For this review, take the finished solid that the model builds, in its own axes (mm). A direction names the side the tool comes from. Coordinates: 2 decimals unless noted, no trailing zeros. Order: outer loops, then holes, each group sorted by start corner. A loop starts at its lowest first (then second) coordinate and runs counter-clockwise, first axis right, second up.
Autodesk Inventor part; units mm, degrees
ref_plane "YZ Plane" through (0, 0, 0) normal (1, 0, 0) x (0, 1, 0)
ref_plane "XZ Plane" through (0, 0, 0) normal (0, 1, 0) x (-1, 0, 0)
ref_plane "XY Plane" through (0, 0, 0) normal (0, 0, 1) x (1, 0, 0)
sketch "Sketch1" plane through (0, 0, 0) normal (0, 1, 0) x (-1, 0, 0)
  line L0 (0, 74.2932) -> (20.6375, 74.2932)
  line L1 (20.6375, 74.2932) -> (20.6375, 45.7421)
  line L2 (13.589, 67.9432) -> (0, 67.9432)
  line L3 (16.6624, -52.7068) -> (20.6375, -52.7068)
  line L4 (20.6375, -52.7068) -> (20.6375, 45.7421)
  line L5 (16.6624, -52.7068) -> (16.6624, -78.1068)
  line L6 (16.6624, -78.1068) -> (13.589, -78.1068)
  line L7 (13.589, -78.1068) -> (13.589, 67.9432)
  line L8 (0, 68.4776) -> (0, -51.9613) construction
  line L9 (13.589, 67.9432) -> (13.589, 74.2932)
  point P0 (0, 0)
  dimension "d0" = 20.6375
  dimension "d1" = 127
  dimension "d2" = 6.35
  dimension "d3" = 16.6624
  dimension "d4" = 13.589
  dimension "d12" = 25.4
  dimension "d19" = 3.0734
revolve "Revolution1" add sketch "Sketch1" angle 360 about axis through (0, 0, 68.4776) along (0, 0, -1)
thread "Thread1"
chamfer "Chamfer2" distance 1.27 angle 45 1 edges at (20.6375, 0, -52.7068)
chamfer "Chamfer3" distance 1.27 angle 45 1 edges at (20.6375, 0, 74.2932)
properties part number "EndHilt" material "Aluminum 6061"
1. To check wall thickness, follow L1, parallel to Y at x = 0, z = 0.5; L2, parallel to Z at x = 11, y = 14; L3, parallel to X at y = 6, z = -23.5. State the ranges of each line that lie inside material, in increasing order.
Answer below:
L1: y = -20.64 to -13.59, 13.59 to 20.64
L2: z = -52.71 to 74.29
L3: x = -19.75 to -12.19, 12.19 to 19.75
2. The part is to be moulded in two halves that separate along Y. For faces 1 (the face through (4.474, -20.147, 9.922)), 2 (the face through (14, 0, -78.107)), 3 (the face through (-12.96, -4.08, -0.84)), say which applies: +Y half, -Y half, draft (parallel to the pull), parting line (faces both ways), or undercut.
Answer below:
face 1: parting line
face 2: draft
face 3: undercut
3. Clearance check with flat-ended pins moving along their axes: pin 1 Ø3 at (y, z) = (4.5, 52) entering from -X; pin 2 Ø1 at (x, z) = (2.5, 11.5) entering from -Y; pin 3 Ø1.5 at (y, z) = (-7.5, -32) entering from -X. State where each tip first meets the part, or that it passes through.
Answer below:
pin 1: stops at x = -20.42
pin 2: stops at y = -20.54
pin 3: stops at x = -19.5
4. Machinability: for faces 4 (the face through (13.2, -4, 74.293)), 5 (the face through (-6, 16, -52.707)), which of the approach directions +Z, -Z, +X, -X, +Y, -Y give a long, thin tool a straight path to every point of the face, cutting with its end or side? Answer none if there is none.
Answer below:
face 4: +Z, +X, -X, +Y, -Y
face 5: -Z
5. Take a section at A-A, the plane y = 0. Give the boundary of the cut face in (x, z).
Answer below:
outline: (-20.64, -51.44) - (-19.37, -52.71) - (-16.66, -52.71) - (-16.66, -78.11) - (-13.59, -78.11) - (-13.59, 74.29) - (-19.37, 74.29) - (-20.64, 73.02) - close; (13.59, -78.11) - (16.66, -78.11) - (16.66, -52.71) - (19.37, -52.71) - (20.64, -51.44) - (20.64, 73.02) - (19.37, 74.29) - (13.59, 74.29) - close
6. Take a section at C-C, the plane z = -65. Give the boundary of the cut face in (x, y).
Answer below:
outline: circle Ø33.32 at (0, 0); hole circle Ø27.18 at (0, 0)
7. Take a section at D-D, the plane z = 61. Give the boundary of the cut face in (x, y) (1 decimal), plus the area to 3 significant figures.
Answer below:
outline: circle Ø41.3 at (0, 0); hole circle Ø27.2 at (0, 0)
area: 758 mm2
